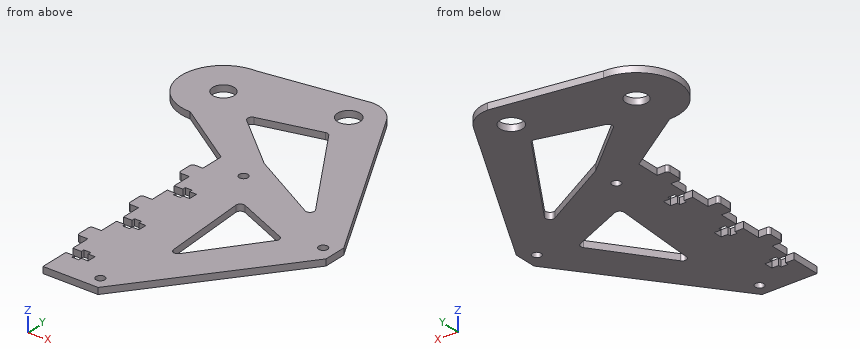
from build123d import *

# Parameters (mm, degrees)
SKETCH_1_R      = 5.0225
SKETCH_1_R_2    = 2.05
SKETCH_1_R_3    = 5.25
EXTRUDE_1_DEPTH = 3
FILLET_1_R      = 2
FILLET_2_R      = 1.3


with BuildPart() as part:
    # 草图1 → 凸台-拉伸1 (new body)
    with BuildSketch(Plane.XY):
        with BuildLine():
            Line((298.545628784, -83.894391363), (298.545628784, -92.841778663))
            Line((298.545628784, -92.841778663), (302.545628784, -92.841778663))
            Line((302.545628784, -92.841778663), (302.545628784, -91.391778663))
            Line((302.545628784, -91.391778663), (305.745628784, -91.391778663))
            Line((305.745628784, -91.391778663), (305.745628784, -92.841778663))
            Line((305.745628784, -92.841778663), (308.945628784, -92.841778663))
            Line((308.945628784, -92.841778663), (308.945628784, -96.941778663))
            Line((308.945628784, -96.941778663), (305.745628784, -96.941778663))
            Line((305.745628784, -96.941778663), (305.745628784, -98.391778663))
            Line((305.745628784, -98.391778663), (302.545628784, -98.391778663))
            Line((302.545628784, -98.391778663), (302.545628784, -96.941778663))
            Line((302.545628784, -96.941778663), (298.545628784, -96.941778663))
            Line((298.545628784, -96.941778663), (298.545628784, -105.894391358))
            Line((298.545628784, -105.894391358), (293.545628784, -105.894391358))
            Line((293.545628784, -105.894391358), (293.545628784, -113.894391358))
            Line((293.545628784, -113.894391358), (298.545628784, -113.894391358))
            Line((298.545628784, -113.894391358), (298.545628784, -122.847004054))
            Line((298.545628784, -122.847004054), (302.545628784, -122.847004054))
            Line((302.545628784, -122.847004054), (302.545628784, -121.397004054))
            Line((302.545628784, -121.397004054), (305.745628784, -121.397004054))
            Line((305.745628784, -121.397004054), (305.745628784, -122.847004054))
            Line((305.745628784, -122.847004054), (308.945628784, -122.847004054))
            Line((308.945628784, -122.847004054), (308.945628784, -126.947004054))
            Line((308.945628784, -126.947004054), (305.745628784, -126.947004054))
            Line((305.745628784, -126.947004054), (305.745628784, -128.397004054))
            Line((305.745628784, -128.397004054), (302.545628784, -128.397004054))
            Line((302.545628784, -128.397004054), (302.545628784, -126.947004054))
            Line((302.545628784, -126.947004054), (298.545628784, -126.947004054))
            Line((298.545628784, -126.947004054), (298.545628784, -140.447004054))
            Line((298.545628784, -140.447004054), (324.188862368, -140.447004054))
            Line((324.188862368, -140.447004054), (376.358604426, -71.946984141))
            Line((376.358604426, -71.946984141), (376.358604426, -61.391778668))
            Line((376.358604426, -61.391778668), (328.961754808, 24.094724856))
            ThreePointArc((328.961754808, 24.094724856), (323.822689813, 29.369350164), (316.717741365, 31.306195206))
            Line((316.717741365, 31.306195206), (268.536959304, 24.041593685))
            ThreePointArc((268.536959304, 24.041593685), (248.891566772, 4.396186988), (268.536987634, -15.249191379))
            Line((268.536987634, -15.249191379), (298.545628784, -35.096984141))
            Line((298.545628784, -35.096984141), (298.545628784, -45.889165972))
            Line((298.545628784, -45.889165972), (293.545628784, -45.889165972))
            Line((293.545628784, -45.889165972), (293.545628784, -53.889165972))
            Line((293.545628784, -53.889165972), (298.545628784, -53.889165972))
            Line((298.545628784, -53.889165972), (298.545628784, -62.841778668))
            Line((298.545628784, -62.841778668), (302.545628784, -62.841778668))
            Line((302.545628784, -62.841778668), (302.545628784, -61.391778668))
            Line((302.545628784, -61.391778668), (305.745628784, -61.391778668))
            Line((305.745628784, -61.391778668), (305.745628784, -62.841778668))
            Line((305.745628784, -62.841778668), (308.945628784, -62.841778668))
            Line((308.945628784, -62.841778668), (308.945628784, -66.941778668))
            Line((308.945628784, -66.941778668), (305.745628784, -66.941778668))
            Line((305.745628784, -66.941778668), (305.745628784, -68.391778668))
            Line((305.745628784, -68.391778668), (302.545628784, -68.391778668))
            Line((302.545628784, -68.391778668), (302.545628784, -66.941778668))
            Line((302.545628784, -66.941778668), (298.545628784, -66.941778668))
            Line((298.545628784, -66.941778668), (298.545628784, -75.894391363))
            Line((298.545628784, -75.894391363), (293.545628784, -75.894391363))
            Line((293.545628784, -75.894391363), (293.545628784, -83.894391363))
            Line((293.545628784, -83.894391363), (298.545628784, -83.894391363))
        make_face()
        with Locations((268.536959304, 4.396201153)):
            Circle(SKETCH_1_R, mode=Mode.SUBTRACT)
        with Locations((320.545628784, -134.447004054)):
            Circle(SKETCH_1_R_2, mode=Mode.SUBTRACT)
        with Locations((370.358604426, -65.946984141)):
            Circle(SKETCH_1_R_2, mode=Mode.SUBTRACT)
        with Locations((313.936987634, -41.346984141)):
            Circle(SKETCH_1_R_2, mode=Mode.SUBTRACT)
        with Locations((316.717741365, 17.306195206)):
            Circle(SKETCH_1_R_3, mode=Mode.SUBTRACT)
        Polygon((354.947285032, -70.136765586), (328.579617375, -106.396108383), (325.08144343, -57.115165973), align=None, mode=Mode.SUBTRACT)
        Polygon((318.527528456, 3.423664072), (285.781281912, -5.015216674), (313.936947803, -29.165661305), (354.9472452, -52.015830841), align=None, mode=Mode.SUBTRACT)
    extrude(amount=EXTRUDE_1_DEPTH)

    # 圆角1
    fillet_1_edges = [part.edges().sort_by_distance(p)[0] for p in [
        (354.9472452, -52.015830841, 1.5),
        (318.527528456, 3.423664072, 1.5),
        (285.781281912, -5.015216674, 1.5),
        (313.936947803, -29.165661305, 1.5),
        (354.947285032, -70.136765586, 1.5),
        (325.08144343, -57.115165973, 1.5),
        (328.579617375, -106.396108383, 1.5),
    ]]
    fillet(fillet_1_edges, radius=FILLET_1_R)

    # 圆角2
    fillet_2_edges = [part.edges().sort_by_distance(p)[0] for p in [
        (293.545628784, -83.894391363, 1.5),
        (293.545628784, -75.894391363, 1.5),
        (293.545628784, -53.889165972, 1.5),
        (293.545628784, -45.889165972, 1.5),
        (293.545628784, -113.894391358, 1.5),
        (293.545628784, -105.894391358, 1.5),
    ]]
    fillet(fillet_2_edges, radius=FILLET_2_R)


solid = part.part
Here's how the part is built. I have some questions about the finished solid (model axes, mm). Give positions to 0.01 mm unless a question says otherwise; leave off trailing zeros. Loops run counter-clockwise (first coordinate to the right, second up) from the corner with the lowest first, then second, coordinate; pieces in that order, holes last. Notation, with made-up numbers: (-0.5, 24) -> (13.5, 24) arc R20 cw to (13.5, 34) -> close; hole circle Ø4 at (61.25, 8). An arc over 180 degrees is marked (long way). One line per item, written item: value.
Q1. Suppose I cut it at D-D on z = 1.3. State how many separate pieces and enclosed holes the cut face has, then the cut area to 3 significant figures.
Answers follow:
separate pieces: 1
enclosed holes: 7
area: 9,140 mm^2
Q2. I'm going to push flat-ended pins straight in: pin 1 Ø0.9 at (x, z) = (307.5, 1.5) entering from +Y; pin 2 Ø3 at (x, y) = (322, -5) entering from +Z; pin 3 Ø0.9 at (y, z) = (-125.5, 2) entering from -X; pin 4 Ø0.9 at (x, z) = (296, 1) entering from +Y. Where does each tip first touch, or does it pass through?
Answers follow:
pin 1: y = 29.98
pin 2: through
pin 3: x = 308.95
pin 4: y = 28.25
Q3. Suppose I cut it at A-A on x = 345. Please give me the cut outline in (y, z), then the cut area to 3 significant figures.
Answers follow:
outline: (-113.12, 0) -> (-83.82, 0) -> (-83.82, 3) -> (-113.12, 3) -> close; (-65.8, 0) -> (-46.47, 0) -> (-46.47, 3) -> (-65.8, 3) -> close; (-36.87, 0) -> (-4.83, 0) -> (-4.83, 3) -> (-36.87, 3) -> close
area: 242 mm^2
Q4. If I drill on line 1 along Y through (x, z) = (330, 0.2); line 2 along Y through (x, z) = (305, 1.25); line 3 along Y through (x, z) = (301, 0.75), over which ranges is the centre line in solid material (lowest first)?
Answers follow:
line 1: -132.82 to -102.78, -59.26 to -38.12, -14.04 to 22.22
line 2: -140.45 to -128.4, -121.4 to -98.39, -91.39 to -68.39, -61.39 to -21.5, -0.06 to 29.54
line 3: -140.45 to -126.95, -122.85 to -96.94, -92.84 to -66.94, -62.84 to -18.07, -1.09 to 28.94
Q5. Suppose I cut it at C-C on x = 271. Please give me the cut outline in (y, z), then the cut area to 3 significant figures.
Answers follow:
outline: (-16.88, 0) -> (0.02, 0) -> (0.02, 3) -> (-16.88, 3) -> close; (8.77, 0) -> (24.41, 0) -> (24.41, 3) -> (8.77, 3) -> close
area: 97.6 mm^2
Q6. Suppose I cut it at B-B on y = 7. Please give me the cut outline in (x, z), then the cut area to 3 significant figures.
Answers follow:
outline: (249.06, 0) -> (264.24, 0) -> (264.24, 3) -> (249.06, 3) -> close; (272.83, 0) -> (338.44, 0) -> (338.44, 3) -> (272.83, 3) -> close
area: 242 mm^2
